For this review, use the dimensioned drawing (mm, ordinates from the lowest corner) and the shaded views. A direction names the side the tool comes from. Round coordinates to 2 decimals unless told otherwise and drop trailing zeros. Order: outer loops, then holes, each group sorted by start corner. A loop starts at its lowest first (then second) coordinate and runs counter-clockwise, first axis right, second up. Notation, with made-up numbers: (70, 72) - (103, 72) arc R9 cw to (103, 88) - close; hole circle Ø6 at (51.5, 81). An arc over 180 degrees is marked (long way). Use CSV: the item, a comma, the result in double quotes. Start each with the question number.
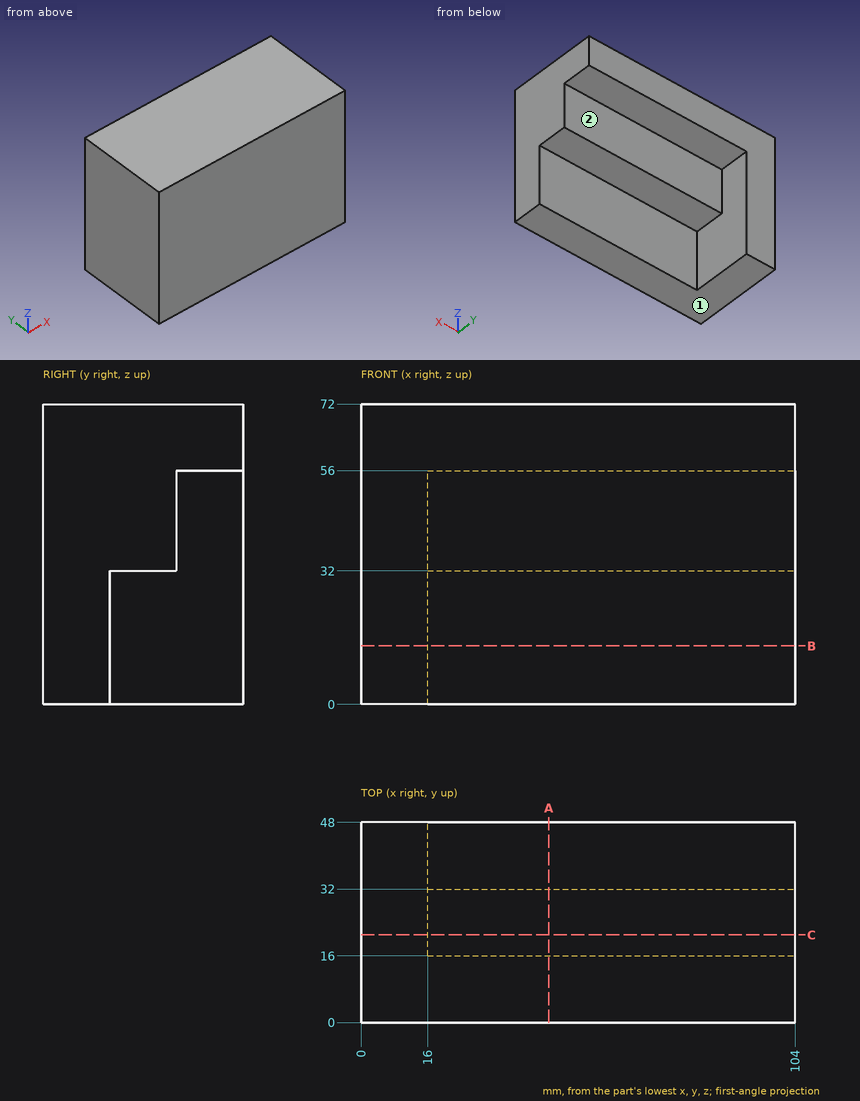
Q1. Take a section at B-B (z = 14). State the section outline as (x, y) points.
Q2. Clearance check with flat-ended pins moving along their axes: pin 1 (9.5 mm diameter, centred on x = 58, z = 15, fed in from +Y); pin 2 (9.5 mm diameter, centred on y = 36, z = 20, fed in from +X); pin 3 (13 mm diameter, centred on x = 54, y = 39.5, fed in from -Z). State where each tip first meets the part, or that it passes through.
Q3. Take a section at A-A (x = 45). State the section outline as (y, z) points, plus the area to 3 significant figures.
Q4. Take a section at C-C (y = 21). State the section outline as (x, z) points, plus the area to 3 significant figures.
Q5. For L1, parallel to Z at x = 72, y = 42; L2, parallel to Y at x = 73, z = 47; L3, parallel to Z at x = 53, y = 28, list the stretches that pass through material, from the lowest coordinate up. Write a range as [from, to].
Q6. Tool access review of the marked faces 1 and 2: name each direction out of +Z, -Z, +X, -X, +Y, -Y from which nothing blocks a thin tool from reaching the whole face with its end or side.
Findings below:
1,outline,"(0, 0) - (104, 0) - (104, 16) - (16, 16) - (16, 48) - (0, 48) - close"
2,pin 1,"stops at y = 16"
2,pin 2,"stops at x = 16"
2,pin 3,"stops at z = 56"
3,outline,"(0, 0) - (16, 0) - (16, 32) - (32, 32) - (32, 56) - (48, 56) - (48, 72) - (0, 72) - close"
3,area,"2,050 mm^2"
4,outline,"(0, 0) - (16, 0) - (16, 32) - (104, 32) - (104, 72) - (0, 72) - close"
4,area,"4,670 mm^2"
5,L1,"z = [56, 72]"
5,L2,"y = [0, 32]"
5,L3,"z = [32, 72]"
6,face 1,"-Z, +X, -X, +Y, -Y"
6,face 2,"-Z, +X, +Y"
